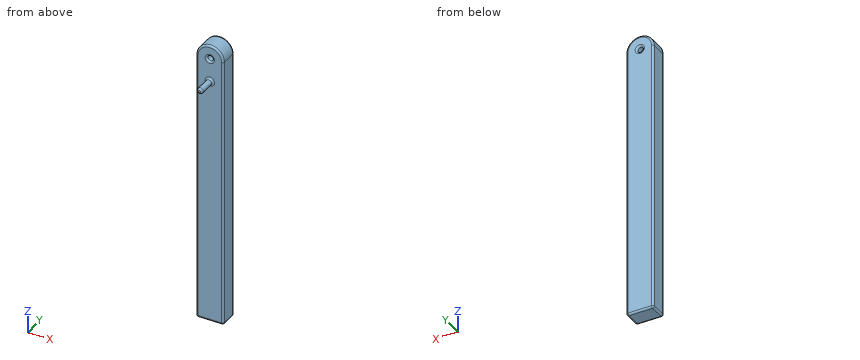
from build123d import *

# Parameters (mm, degrees)
F0_R     = 3.96875
F1_DEPTH = 50.8
F2_DEPTH = 25.4
F3_R     = 2.54


with BuildPart() as f1:
    # F0 (on Front) → F1 (new body)
    with BuildSketch(Plane.XZ):
        with Locations((19.05, 348.1435775757)):
            Circle(F0_R)
    extrude(amount=F1_DEPTH)

    # F0 (on Front) → F2 (join)
    with BuildSketch(Plane.XZ):
        with BuildLine():
            Line((0, 381), (0, 0))
            Line((0, 0), (38.1, 0))
            Line((38.1, 0), (38.1, 381))
            ThreePointArc((38.1, 381), (19.05, 400.05), (0, 381))
        make_face()
        with Locations((19.05, 348.1435775757)):
            Circle(F0_R, mode=Mode.SUBTRACT)
        with Locations((19.05, 381)):
            Circle(F0_R, mode=Mode.SUBTRACT)
    extrude(amount=F2_DEPTH)

    # F3
    f3_edges = [f1.edges().sort_by_distance(p)[0] for p in [
        (15.08125, -25.4, 348.143578),
        (23.01875, -38.1, 348.143578),
        (15.08125, -50.8, 348.143578),
        (19.05, -25.4, 400.05),
        (0, -25.4, 190.5),
        (19.05, -25.4, 0),
        (38.1, -25.4, 190.5),
        (15.08125, -25.4, 381),
        (38.1, -12.7, 381),
        (0, -12.7, 381),
        (19.05, 0, 400.05),
        (0, -12.7, 0),
        (0, 0, 190.5),
        (23.01875, -12.7, 381),
        (15.08125, 0, 381),
        (38.1, -12.7, 0),
        (38.1, 0, 190.5),
        (19.05, 0, 0),
    ]]
    fillet(f3_edges, radius=F3_R)


solid = f1.part
Part model, mm, in its own coordinate system. Give positions to 0.01 mm unless a question says otherwise; leave off trailing zeros. Order: outer loops, then holes, each group sorted by start corner. A loop starts at its lowest first (then second) coordinate and runs counter-clockwise, first axis right, second up. Notation, with made-up numbers: (28, 32) - (50, 32) arc R17 cw to (50, 42) - close; hole circle Ø7 at (-37, 49.25). An arc over 180 degrees is marked (long way). Use a Markdown table: item, result.
1) Flat gauge pins, fed straight in: P1, Ø8, axis at x = 21.5, y = -42, coming from the -Z side; P2, Ø10, axis at x = 20.5, z = 157, coming from the -Y side; P3, Ø4, axis at x = 14, y = -13, coming from the +Z side. Where does each tip first touch, or does it go through?
Checked values:
| item | result |
|---|---|
| P1 | z = 344.17 |
| P2 | y = -25.4 |
| P3 | z = 399.8 |
2) Probe L1, parallel to X at y = -13.5, z = 381; L2, parallel to Z at x = 19.05, y = -11.5; L3, parallel to Y at x = 24, z = 195. List the from-to ranges inside material, lowest first. Write a range as from..to.
Checked values:
| item | result |
|---|---|
| L1 | 0..15.08, 23.02..38.1 |
| L2 | 0..377.03, 384.97..400.05 |
| L3 | -25.4..0 |
3) Saw through at A-A on y = -33. List the corners of the cut face in (x, z).
Checked values:
| item | result |
|---|---|
| outline | circle Ø7.94 at (19.05, 348.14) |
